from build123d import *

# Parameters (mm, degrees)
SKETCH1_W       = 35
SKETCH1_H       = 12
EXTRUDE1_DEPTH  = 6
SKETCH2_W       = 6
SKETCH2_H       = 12
EXTRUDE2_DEPTH  = 4
SKETCH3_R       = 1.5
EXTRUDE3_DEPTH  = 2
SKETCH4_R       = 1.6
EXTRUDE4_DEPTH  = 6
SKETCH7_W       = 15
SKETCH7_H       = 12
EXTRUDE6_DEPTH  = 2.5
SKETCH8_W       = 27
SKETCH8_H       = 12
EXTRUDE7_DEPTH  = 1.5
SKETCH9_W       = 4.5
SKETCH9_H       = 12
EXTRUDE8_DEPTH  = 17.26
SKETCH10_W      = 8
SKETCH10_H      = 2
EXTRUDE9_DEPTH  = 12
SKETCH12_R      = 1.5
EXTRUDE10_DEPTH = 2


with BuildPart() as part:
    # Sketch1 → Extrude1 (new body)
    with BuildSketch(Plane.XY):
        Rectangle(SKETCH1_W, SKETCH1_H)
    extrude(amount=EXTRUDE1_DEPTH)

    # Sketch2 → Extrude2 (cut)
    with BuildSketch(Plane.XY.offset(6)):
        with Locations((-14.5, 0)):
            Rectangle(SKETCH2_W, SKETCH2_H)
    extrude(amount=-EXTRUDE2_DEPTH, mode=Mode.SUBTRACT)

    # Sketch3 → Extrude3 (cut)
    with BuildSketch(Plane.XY.offset(2)):
        with Locations((-14.5, 3)):
            Circle(SKETCH3_R)
        with Locations((-14.5, -3)):
            Circle(SKETCH3_R)
    extrude(amount=-EXTRUDE3_DEPTH, mode=Mode.SUBTRACT)

    # Sketch4 → Extrude4 (cut)
    with BuildSketch(Plane.XY.offset(6)):
        with Locations((9.88, 0)):
            Circle(SKETCH4_R)
    extrude(amount=-EXTRUDE4_DEPTH, mode=Mode.SUBTRACT)

    # Sketch7 → Extrude6 (cut)
    with BuildSketch(Plane.XY.offset(6)):
        with Locations((10, 0)):
            Rectangle(SKETCH7_W, SKETCH7_H)
    extrude(amount=-EXTRUDE6_DEPTH, mode=Mode.SUBTRACT)

    # Sketch8 → Extrude7 (cut)
    with BuildSketch(Plane(origin=(0, 0, 0), x_dir=(-1, 0, 0), z_dir=(0, 0, -1))):
        with Locations((-4, 0)):
            Rectangle(SKETCH8_W, SKETCH8_H)
    extrude(amount=-EXTRUDE7_DEPTH, mode=Mode.SUBTRACT)

    # Sketch9 → Extrude8 (add)
    with BuildSketch(Plane(origin=(17.5, 0, 0), x_dir=(0, 0, -1), z_dir=(1, 0, 0))):
        with Locations((-3.75, 0)):
            Rectangle(SKETCH9_W, SKETCH9_H)
    extrude(amount=EXTRUDE8_DEPTH)

    # Sketch10 → Extrude9 (add)
    with BuildSketch(Plane(origin=(0, 6, 0), x_dir=(1, 0, 0), z_dir=(0, 1, 0))):
        with Locations((36.76, -0.5)):
            Rectangle(SKETCH10_W, SKETCH10_H)
    extrude(amount=-EXTRUDE9_DEPTH)

    # Sketch12 → Extrude10 (cut)
    with BuildSketch(Plane.XY.offset(1.5)):
        with Locations((37.76, 3)):
            Circle(SKETCH12_R)
        with Locations((37.76, -3)):
            Circle(SKETCH12_R)
    extrude(amount=-EXTRUDE10_DEPTH, mode=Mode.SUBTRACT)


solid = part.part
For this review, take the finished solid that the model builds, in its own axes (mm). A direction names the side the tool comes from. Coordinates: 2 decimals unless noted, no trailing zeros. Loops run counter-clockwise (first coordinate to the right, second up) from the corner with the lowest first, then second, coordinate; pieces in that order, holes last. Notation, with made-up numbers: (-10.5, 53.25) - (-3.5, 53.25) arc R25 cw to (-3.5, 90.25) - close; hole circle Ø6 at (89, -24). An arc over 180 degrees is marked (long way). Use a Markdown table: item, result. Add a question column.
Item 1: For line 1 (Y direction, x = -14.5, z = 1.3); line 2 (X direction, y = -5, z = 3.75); line 3 (Y direction, x = 9.88, z = 2.25), list the stretches that pass through material, from the lowest coordinate up.
Item 2: We need section D-D (y = -3). Give the boundary of the cut face in (x, z), and give its area (3 significant figures).
Item 3: Insertion check: pin 1 Ø4 at (x, y) = (9.88, 0) entering from -Z; pin 2 Ø2.5 at (x, y) = (-14.5, -2.5) entering from -Z; pin 3 Ø3 at (y, z) = (1, 4) entering from -X. Each pin has a flat end and moves straight along its axis. Give the tip position at first contact, or say it passes through.
Item 4: Tool access review of faces 4 (the face through (11.3, 1.2, 1.5)), 5 (the face through (39.19, 3.45, 0.51)), 6 (the face through (2.5, 0, 5)), 7 (the face through (-11.5, 0, 4)), 8 (the face through (38, 0, 1.5)): name each direction out of +Z, -Z, +X, -X, +Y, -Y from which nothing blocks a thin tool from reaching the whole face with its end or side.
Item 5: We need section A-A (x = 9.88). Give the boundary of the cut face in (y, z), and give its area (3 significant figures).
Item 6: Mouldability with a two-part tool opening along Y and no side actions: class faces 1 (the face through (-16, -3, 1)), 2 (the face through (11, 6, 3)), 3 (the face through (-15, 0, 2)) as pulls with the +Y half, pulls with the -Y half, needs draft (parallel to the pull), parting line crosses it, or undercut.
Item 7: We need section B-B (y = 0). Give the boundary of the cut face in (x, z), and give its area (3 significant figures).
Item 8: We need section C-C (z = 5). Give the boundary of the cut face in (x, y).
Results list:
| question | item | result |
|---|---|---|
| 1 | line 1 | y = -6 to -4.5, -1.5 to 1.5, 4.5 to 6 |
| 1 | line 2 | x = -11.5 to 2.5, 17.5 to 34.76 |
| 1 | line 3 | y = -6 to -1.6, 1.6 to 6 |
| 2 | outline | (-17.5, 0) - (-16, 0) - (-16, 2) - (-17.5, 2) - close; (-13, 0) - (-9.5, 0) - (-9.5, 1.5) - (32.76, 1.5) - (32.76, -0.5) - (36.26, -0.5) - (36.26, 1.5) - (34.76, 1.5) - (34.76, 6) - (17.5, 6) - (17.5, 3.5) - (2.5, 3.5) - (2.5, 6) - (-11.5, 6) - (-11.5, 2) - (-13, 2) - close; (39.26, -0.5) - (40.76, -0.5) - (40.76, 1.5) - (39.26, 1.5) - close |
| 2 | area | 190 mm^2 |
| 3 | pin 1 | stops at z = 1.5 |
| 3 | pin 2 | stops at z = 0 |
| 3 | pin 3 | stops at x = -11.5 |
| 4 | face 4 | -Z, +Y, -Y |
| 4 | face 5 | +Z, -Z |
| 4 | face 6 | +Z, +Y, -Y |
| 4 | face 7 | +Z, -X, +Y, -Y |
| 4 | face 8 | +Z, +X, +Y, -Y |
| 5 | outline | (-6, 1.5) - (-1.6, 1.5) - (-1.6, 3.5) - (-6, 3.5) - close; (1.6, 1.5) - (6, 1.5) - (6, 3.5) - (1.6, 3.5) - close |
| 5 | area | 17.6 mm^2 |
| 6 | face 1 | undercut |
| 6 | face 2 | pulls with the +Y half |
| 6 | face 3 | needs draft |
| 7 | outline | (-17.5, 0) - (-9.5, 0) - (-9.5, 1.5) - (8.28, 1.5) - (8.28, 3.5) - (2.5, 3.5) - (2.5, 6) - (-11.5, 6) - (-11.5, 2) - (-17.5, 2) - close; (11.48, 1.5) - (32.76, 1.5) - (32.76, -0.5) - (40.76, -0.5) - (40.76, 1.5) - (34.76, 1.5) - (34.76, 6) - (17.5, 6) - (17.5, 3.5) - (11.48, 3.5) - close |
| 7 | area | 195 mm^2 |
| 8 | outline | (-11.5, -6) - (2.5, -6) - (2.5, 6) - (-11.5, 6) - close; (17.5, -6) - (34.76, -6) - (34.76, 6) - (17.5, 6) - close |
